```python
from build123d import *

# Parameters (mm, degrees)
SKETCH_1_R          = 3
EXTRUDE_1_DEPTH     = 1
SKETCH_3_R          = 1
CUT_EXTRUDE_1_DEPTH = 5.358898944


with BuildPart() as part:
    # 草图1 → 凸台-拉伸1 (new body)
    with BuildSketch(Plane.XY):
        Circle(SKETCH_1_R)
    extrude(amount=EXTRUDE_1_DEPTH)

    # 草图2 → 切除-旋转1 (revolve, cut)
    with BuildSketch(Plane(origin=(0, 0, 0), x_dir=(1, 0, 0), z_dir=(0, 1, 0))):
        with BuildLine():
            Line((1.5, 0), (2.5, 0))
            ThreePointArc((2.5, 0), (2, -0.5), (1.5, 0))
        make_face()
    revolve(axis=Axis((0, 0, 1), (0, 0, -1)), mode=Mode.SUBTRACT)

    # 草图3 → 切除-拉伸1 (cut, through all)
    with BuildSketch(Plane(origin=(0, 0, 0), x_dir=(-1, 0, 0), z_dir=(0, 0, -1))):
        Circle(SKETCH_3_R)
    extrude(amount=-CUT_EXTRUDE_1_DEPTH, mode=Mode.SUBTRACT)


solid = part.part
```
Source: CAD feature listing. Evaluate the final solid. Frame: model axes, mm. Coordinates: 2 decimals unless noted, no trailing zeros. Write each loop counter-clockwise with the first axis right and the second up, starting at its lowest first coordinate (ties: lowest second). Pieces come first, ordered by that corner, then holes. Notation, with made-up numbers: M 43,27 L 51,27 A27 cw 51,46 Z; hole C -14,23.25 d2. An arc over 180 degrees is marked long. Answer as a JSON object with one key per item and string values.
1. Cut plane D-D on z = 0.85. Output: boundary loops of the cut face in (x, y), plus the area to 3 significant figures.
Evaluation:
{"outline": "C 0,0 d6; hole C 0,0 d2", "area": "25.1 mm^2"}
2. Ray query, L1, parallel to Y at x = 0, z = 0.65; L2, parallel to Z at x = -1.75, y = -1; L3, parallel to X at y = 1.85, z = 0.1. Return the intervals inside material, ascending.
Evaluation:
{"L1": "-3 to -1, 1 to 3", "L2": "0.5 to 1", "L3": "-2.36 to -1.67, 1.67 to 2.36"}
3. Cut plane A-A on x = 0. Output: boundary loops of the cut face in (y, z).
Evaluation:
{"outline": "M -3,0 L -2.5,0 A0.5 cw -1.5,0 L -1,0 L -1,1 L -3,1 Z; M 1,0 L 1.5,0 A0.5 cw 2.5,0 L 3,0 L 3,1 L 1,1 Z"}
4. Cut plane C-C on z = 0.35. Output: boundary loops of the cut face in (x, y), plus the area to 3 significant figures.
Evaluation:
{"outline": "C 0,0 d6; C 0,0 d3.29; hole C 0,0 d4.71; hole C 0,0 d2", "area": "16.2 mm^2"}
5. Draft query along Y for faces 1 (the cylindrical face through (0.217, -0.976, 0.493)), 2 (the flat face through (-1, 1, 1)), 3 (the cylindrical face through (-3, 0.1, 0.5)). Return one class per face: released by +Y, released by -Y, zero draft, split by the parting line, or undercut.
Evaluation:
{"face 1": "undercut", "face 2": "zero draft", "face 3": "split by the parting line"}
